from build123d import *

# Parameters (mm, degrees)
BOSS_EXTRUDE1_DEPTH = 30
SKETCH2_R           = 1.5
CUT_EXTRUDE1_DEPTH  = 39.065732621
FILLET1_R           = 3
SKETCH3_R           = 1.5
CUT_EXTRUDE2_DEPTH  = 30


with BuildPart() as part:
    # Sketch1 → Boss-Extrude1 (new body)
    with BuildSketch(Plane.XY):
        Polygon((0, 0), (15, 0), (15, 18), (0, 18), (0, 16), (13, 16), (13, 2), (0, 2), align=None)
    extrude(amount=BOSS_EXTRUDE1_DEPTH)

    # Sketch2 → Cut-Extrude1 (cut, through all)
    with BuildSketch(Plane(origin=(0, 18, 0), x_dir=(1, 0, 0), z_dir=(0, 1, 0))):
        with Locations(Location((4, -5, 0), (0, 0, 270))):
            Circle(SKETCH2_R)
        with Locations(Location((4, -25, 0), (0, 0, 270))):
            Circle(SKETCH2_R)
    extrude(amount=-CUT_EXTRUDE1_DEPTH, mode=Mode.SUBTRACT)

    # Fillet1
    fillet1_edges = [part.edges().sort_by_distance(p)[0] for p in [
        (0, 1, 0),
        (0, 17, 30),
        (0, 1, 30),
        (0, 17, 0),
    ]]
    fillet(fillet1_edges, radius=FILLET1_R)

    # Sketch3 → Cut-Extrude2 (cut)
    with BuildSketch(Plane(origin=(15, 0, 0), x_dir=(0, 0, -1), z_dir=(1, 0, 0))):
        with Locations((-15, 9)):
            Circle(SKETCH3_R)
        with BuildLine():
            ThreePointArc((-4.460075902, 4.4), (-3.5, 9), (-4.460075902, 13.6))
            ThreePointArc((-4.460075902, 13.6), (-6.43484861, 14.374772708), (-7.209621319, 12.4))
            ThreePointArc((-7.209621319, 12.4), (-6.5, 9), (-7.209621319, 5.6))
            ThreePointArc((-7.209621319, 5.6), (-6.43484861, 3.625227292), (-4.460075902, 4.4))
        make_face()
    extrude(amount=-CUT_EXTRUDE2_DEPTH, mode=Mode.SUBTRACT)


solid = part.part
Geometry check sheet. Reference: the model listing, model coordinates, mm. A direction names the side the tool comes from. Give positions to 0.01 mm unless a question says otherwise; leave off trailing zeros. Loops run counter-clockwise (first coordinate to the right, second up) from the corner with the lowest first, then second, coordinate; pieces in that order, holes last.
(1) Release check for a two-part mould opening along Y. For faces 3 (the flat face through (7, 0, 15)), 4 (the cylindrical face through (14, 8.9, 3.5)), 5 (the flat face through (15, 11, 15)) record: released by +Y, released by -Y, zero draft, split by the parting line, or undercut.
From the geometry:
face 3: released by -Y
face 4: undercut
face 5: zero draft
(2) Set-up check for faces 1 (the flat face through (7, 2, 15)), 2 (the flat face through (13.4, 9, 0)): record each of +Z, -Z, +X, -X, +Y, -Y from which the full face is reachable in a straight line by a thin tool's end or side.
From the geometry:
face 1: +Z, -Z, -X
face 2: -Z, +X, -X, +Y, -Y
(3) Thickness scan on L1, parallel to Y at x = 8.5, z = 5.75; L2, parallel to X at y = 1.1, z = 5; L3, parallel to Y at x = 13.4, z = 15. Record the ranges inside material, lowest first.
From the geometry:
L1: y = 0 to 2, 16 to 18
L2: x = 0 to 2.5, 5.5 to 15
L3: y = 0 to 7.5, 10.5 to 18
(4) Section check C-C on y = 9. Record the cut outline in (x, z).
From the geometry:
outline: (13, 0) - (15, 0) - (15, 3.5) - (13, 3.5) - close; (13, 6.5) - (15, 6.5) - (15, 13.5) - (13, 13.5) - close; (13, 16.5) - (15, 16.5) - (15, 30) - (13, 30) - close
(5) Section check D-D on z = 25. Record the cut outline in (x, y), then the cut area to 3 significant figures.
From the geometry:
outline: (0, 0) - (2.5, 0) - (2.5, 2) - (0, 2) - close; (0, 16) - (2.5, 16) - (2.5, 18) - (0, 18) - close; (5.5, 0) - (15, 0) - (15, 18) - (5.5, 18) - (5.5, 16) - (13, 16) - (13, 2) - (5.5, 2) - close
area: 76.0 mm2
(6) Section check A-A on z = 15. Record the cut outline in (x, y).
From the geometry:
outline: (0, 0) - (15, 0) - (15, 7.5) - (13, 7.5) - (13, 2) - (0, 2) - close; (0, 16) - (13, 16) - (13, 10.5) - (15, 10.5) - (15, 18) - (0, 18) - close
(7) Section check B-B on x = 8.5. Record the cut outline in (y, z), then the cut area to 3 significant figures.
From the geometry:
outline: (0, 0) - (2, 0) - (2, 30) - (0, 30) - close; (16, 0) - (18, 0) - (18, 30) - (16, 30) - close
area: 120 mm2
(8) Depth check by flat-ended pin: pin 1 Ø2.5 at (y, z) = (9, 15) entering from -X; pin 2 Ø1 at (y, z) = (8.5, 23.5) entering from -X; pin 3 Ø6.5 at (x, z) = (6.5, 12) entering from -Y. Enter the tip coordinate at first touch or a pass-through.
From the geometry:
pin 1: passes through
pin 2: stops at x = 13
pin 3: stops at y = 0
